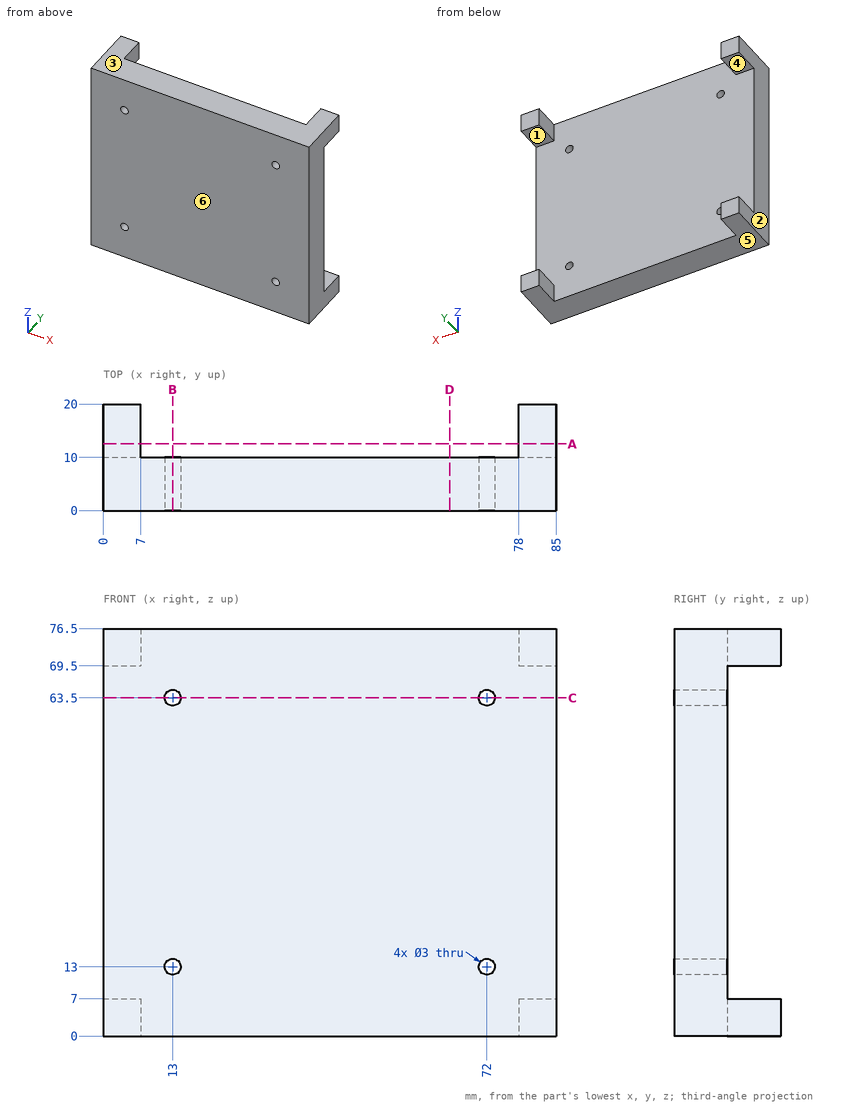
Print and shaded views of the part. All mm, measured from the part's lowest x, y and z. A direction names the side the tool comes from. Round coordinates to 2 decimals unless told otherwise and drop trailing zeros. Write each loop counter-clockwise with the first axis right and the second up, starting at its lowest first coordinate (ties: lowest second). Pieces come first, ordered by that corner, then holes.
(1) 3-axis set-ups, long thin cutter, end or side, ignore diameter. For the marked faces 1 and 2: which of +Z, -Z, +X, -X, +Y, -Y reach the whole face in a straight line?
(2) Mould opens along Z. For the marked faces 3, 4, 5 and 6 say: pulls with the +Z half, pulls with the -Z half, needs draft (parallel to the pull), parting line crosses it, or undercut.
(3) Drop flat-ended pins along their axis: P1, Ø5.5, axis at x = 81.5, y = 14, coming from the -Z side; P2, Ø4, axis at x = 13, z = 63.5, coming from the +Y side. Give the stop position or say it passes through.
(4) Slice it at B-B, the plane x = 13. Write the cut outline in (y, z).
(5) Slice it at A-A, the plane y = 12.5. Write the cut outline in (x, z), and give its area (3 significant figures).
(6) Slice it at D-D, the plane x = 65. Write the cut outline in (y, z), and give its area (3 significant figures).
(7) Slice it at C-C, the plane z = 63.5. Write the cut outline in (x, y), and give its area (3 significant figures).
(8) Probe line 1 along X through (y, z) = (3.25, 63.5); line 2 along Z through (x, y) = (72, 2); line 3 along X through (y, z) = (2.25, 14). List the from-to ranges inside material, lowest first.
From the geometry:
1. face 1: +X, -X, +Y
1. face 2: +Z, -Z, -X, +Y, -Y
2. face 3: pulls with the +Z half
2. face 4: undercut
2. face 5: pulls with the -Z half
2. face 6: needs draft
3. P1: stops at z = 0
3. P2: stops at y = 10
4. outline: (0, 0) - (10, 0) - (10, 11.5) - (0, 11.5) - close; (0, 14.5) - (10, 14.5) - (10, 62) - (0, 62) - close; (0, 65) - (10, 65) - (10, 76.5) - (0, 76.5) - close
5. outline: (0, 0) - (7, 0) - (7, 7) - (0, 7) - close; (0, 69.5) - (7, 69.5) - (7, 76.5) - (0, 76.5) - close; (78, 0) - (85, 0) - (85, 7) - (78, 7) - close; (78, 69.5) - (85, 69.5) - (85, 76.5) - (78, 76.5) - close
5. area: 196 mm2
6. outline: (0, 0) - (10, 0) - (10, 76.5) - (0, 76.5) - close
6. area: 765 mm2
7. outline: (0, 0) - (11.5, 0) - (11.5, 10) - (0, 10) - close; (14.5, 0) - (70.5, 0) - (70.5, 10) - (14.5, 10) - close; (73.5, 0) - (85, 0) - (85, 10) - (73.5, 10) - close
7. area: 790 mm2
8. line 1: x = 0 to 11.5, 14.5 to 70.5, 73.5 to 85
8. line 2: z = 0 to 11.5, 14.5 to 62, 65 to 76.5
8. line 3: x = 0 to 11.88, 14.12 to 70.88, 73.12 to 85
